Autodesk Inventor part; units mm, degrees
ref_plane "YZ Plane" through (0, 0, 0) normal (1, 0, 0) x (0, 1, 0)
ref_plane "XZ Plane" through (0, 0, 0) normal (0, 1, 0) x (-1, 0, 0)
ref_plane "XY Plane" through (0, 0, 0) normal (0, 0, 1) x (1, 0, 0)
sketch "Sketch1" plane through (0, 0, 0) normal (0, 0, 1) x (1, 0, 0)
  ellipse E0 centre (-7.26, 0) end of major axis (-10.02, 0) minor radius 1.8
  ellipse E1 centre (7.26, 0) end of major axis (10.02, 0) minor radius 1.8
  line L0 (11.52, 0) -> (11.52, 3.95)
  line L1 (11.52, 3.95) -> (15.52, 3.95)
  line L2 (15.52, 3.95) -> (15.52, 9.95)
  line L3 (15.52, 9.95) -> (22.84, 9.95)
  line L4 (22.84, 9.95) -> (22.84, 3.95)
  line L5 (22.84, 3.95) -> (26.84, 3.95)
  line L6 (26.84, 3.95) -> (26.84, 0)
  line L7 (11.52, 0) -> (11.52, -3.95)
  line L8 (11.52, -3.95) -> (15.52, -3.95)
  line L9 (15.52, -3.95) -> (15.52, -9.95)
  line L10 (15.52, -9.95) -> (22.84, -9.95)
  line L11 (22.84, -9.95) -> (22.84, -3.95)
  line L12 (22.84, -3.95) -> (26.84, -3.95)
  line L13 (26.84, -3.95) -> (26.84, 0)
  line L14 (-11.52, 0) -> (-11.52, 3.95)
  line L15 (-11.52, 3.95) -> (-15.52, 3.95)
  line L16 (-15.52, 3.95) -> (-15.52, 9.95)
  line L17 (-15.52, 9.95) -> (-22.84, 9.95)
  line L18 (-22.84, 9.95) -> (-22.84, 3.95)
  line L19 (-22.84, 3.95) -> (-26.84, 3.95)
  line L20 (-26.84, 3.95) -> (-26.84, 0)
  line L21 (-11.52, 0) -> (-11.52, -3.95)
  line L22 (-11.52, -3.95) -> (-15.52, -3.95)
  line L23 (-15.52, -3.95) -> (-15.52, -9.95)
  line L24 (-15.52, -9.95) -> (-22.84, -9.95)
  line L25 (-22.84, -9.95) -> (-22.84, -3.95)
  line L26 (-22.84, -3.95) -> (-26.84, -3.95)
  line L27 (-26.84, -3.95) -> (-26.84, 0)
  circle A0 centre (0, -18) radius 8.5
  circle A1 centre (14.5, -29.5) radius 1.5
  circle A2 centre (-14.5, -29.5) radius 1.5
  circle A3 centre (15, -41.5) radius 2
  circle A4 centre (34, -41.5) radius 2
  circle A5 centre (-15, -41.5) radius 2
  circle A6 centre (-34, -41.5) radius 2
  circle A7 centre (-15, -65.5) radius 2
  circle A8 centre (15, -65.5) radius 2
  circle A9 centre (44, -50.5) radius 1.5
  circle A10 centre (-44, -50.5) radius 1.5
  circle A11 centre (0, -57) radius 1.5
  circle A12 centre (20, -57) radius 1.5
  circle A13 centre (34, -57) radius 1.5
  circle A14 centre (-20, -57) radius 1.5
  circle A15 centre (-34, -57) radius 1.5
  circle A16 centre (23.5, -63) radius 1.5
  circle A17 centre (-23.5, -63) radius 1.5
  line L28 (23.84, 13.95) -> (20.76, 13.95)
  line L29 (20.76, 13.95) -> (20.76, 25.98)
  line L30 (20.76, 25.98) -> (23.84, 25.98)
  line L31 (23.84, 25.98) -> (23.84, 13.95)
  line L32 (-23.84, 13.95) -> (-20.76, 13.95)
  line L33 (-20.76, 13.95) -> (-20.76, 25.98)
  line L34 (-20.76, 25.98) -> (-23.84, 25.98)
  line L35 (-23.84, 25.98) -> (-23.84, 13.95)
  circle A18 centre (15, 37) radius 2
  circle A19 centre (15, 62) radius 2
  circle A20 centre (-15, 37) radius 2
  circle A21 centre (-15, 62) radius 2
  circle A22 centre (35, 41.5) radius 1.5
  circle A23 centre (43.5, 50.5) radius 1.5
  circle A24 centre (-35, 41.5) radius 1.5
  circle A25 centre (-43.5, 50.5) radius 1.5
  circle A26 centre (8.5, 55) radius 1.5
  circle A27 centre (23, 55) radius 1.5
  circle A28 centre (-8.5, 55) radius 1.5
  circle A29 centre (-23, 55) radius 1.5
  circle A30 centre (33, 59) radius 1.5
  circle A31 centre (-33, 59) radius 1.5
  circle A32 centre (24, 62) radius 1.5
  circle A33 centre (-24, 62) radius 1.5
  line L36 (-45, 0) -> (-45, 13.95)
  line L37 (-45, 13.95) -> (-41.92, 13.95)
  line L38 (-41.92, 13.95) -> (-41.92, 25.98)
  line L39 (-41.92, 25.98) -> (-45, 25.98)
  line L40 (-45, 25.98) -> (-45, 38.75)
  line L41 (-45, 38.75) -> (-54.4375, 38.75)
  line L42 (-45, 0) -> (-45, -38.75)
  line L43 (-45, -38.75) -> (-54.4375, -38.75)
  line L44 (45, 0) -> (45, 13.95)
  line L45 (45, 13.95) -> (41.92, 13.95)
  line L46 (41.92, 13.95) -> (41.92, 25.98)
  line L47 (41.92, 25.98) -> (45, 25.98)
  line L48 (45, 25.98) -> (45, 38.75)
  line L49 (45, 38.75) -> (54.4375, 38.75)
  line L50 (45, 0) -> (45, -38.75)
  line L51 (45, -38.75) -> (54.4375, -38.75)
  arc A34 (-56.0386, -41.9485) -> (56.0386, -41.9485) centre (0, 0) ccw
  arc A35 (56.0386, 41.9485) -> (-56.0386, 41.9485) centre (0, 0) ccw
  arc A36 (-56.0386, 41.9485) -> (-54.4375, 38.75) centre (-54.4375, 40.75) ccw
  arc A37 (54.4375, 38.75) -> (56.0386, 41.9485) centre (54.4375, 40.75) ccw
  arc A38 (56.0386, -41.9485) -> (54.4375, -38.75) centre (54.4375, -40.75) ccw
  arc A39 (-54.4375, -38.75) -> (-56.0386, -41.9485) centre (-54.4375, -40.75) ccw
  point P0 (-58.2961, 38.75)
  point P1 (-58.2961, -38.75)
  point P2 (58.2961, 38.75)
  point P3 (58.2961, -38.75)
  dimension "d148" = 2
extrude "Extrusion1" add sketch "Sketch1" along normal blind 2.4
properties part number "Part2_Estructura pequeña"
Input: part model. Units: mm. Frame: model coordinates. Give positions to 0.01 mm unless a question says otherwise; leave off trailing zeros. Loops run counter-clockwise (first coordinate to the right, second up) from the corner with the lowest first, then second, coordinate; pieces in that order, holes last. Notation, with made-up numbers: (-25.5, -39.5) -> (-21.5, -39.5) arc R15 cw to (-21.5, -25.5) -> close; hole circle Ø2 at (38, 69). An arc over 180 degrees is marked (long way). Answer as a JSON object with one key per item and string values. Group by question number.
Item 1: Cut plane C-C, the plane y = -21. Return the cut outline in (x, z).
Item 2: Pull-direction query (Y, two-part tool) for faces 1 (the cylindrical face through (-34.11, 57.99, 1.18)), 2 (the flat face through (-1, 1, 0)); classes: released by +Y, released by -Y, zero draft, split by the parting line, or undercut.
Item 3: Cut plane B-B, the plane z = 1.75. State how many separate pieces and enclosed holes the cut face has, and give its area (3 significant figures).
Item 4: Cut plane D-D, the plane y = 31.5. Return the cut outline in (x, z), and give its area (3 significant figures).
Item 5: Cut plane A-A, the plane y = -5.5. Return the cut outline in (x, z).
Item 6: Line query: probe 1 along Y at (x, z) = (20, 1.6); probe 2 along X at (y, z) = (-40.5, 2.2); probe 3 along Y at (x, z) = (6, 1.9). Output: solid intervals per line, ascending.
Item 7: Pin query (flat end, axial travel): P1, Ø1, axis at x = 33.5, z = 2, coming from the +Y side; P2, Ø0.7, axis at y = 21, z = 1, coming from the -X side; P3, Ø3.5, axis at x = 24, y = 62, coming from the -Z side; P4, Ø1.2, axis at x = 13, z = 1, coming from the +Y side. Return the tip coordinate at first contact, or that it passes through.
Checks:
{
 "1": {"outline": "(-45, 0) -> (-7.95, 0) -> (-7.95, 2.4) -> (-45, 2.4) -> close; (7.95, 0) -> (45, 0) -> (45, 2.4) -> (7.95, 2.4) -> close"},
 "2": {"face 1": "undercut", "face 2": "zero draft"},
 "3": {"separate pieces": "1", "enclosed holes": "40", "area": "11,000 mm²"},
 "4": {"outline": "(-45, 0) -> (45, 0) -> (45, 2.4) -> (-45, 2.4) -> close", "area": "216 mm²"},
 "5": {"outline": "(-45, 0) -> (-22.84, 0) -> (-22.84, 2.4) -> (-45, 2.4) -> close; (-15.52, 0) -> (15.52, 0) -> (15.52, 2.4) -> (-15.52, 2.4) -> close; (22.84, 0) -> (45, 0) -> (45, 2.4) -> (22.84, 2.4) -> close"},
 "6": {"probe 1": "y = -67.08 to -58.5, -55.5 to -9.95, 9.95 to 67.08", "probe 2": "x = -56.42 to -35.73, -32.27 to -16.73, -13.27 to 13.27, 16.73 to 32.27, 35.73 to 56.42", "probe 3": "y = -69.74 to -24.02, -11.98 to -1.6, 1.6 to 69.74"},
 "7": {"P1": "stops at y = 61.73", "P2": "stops at x = -41.92", "P3": "stops at z = 0", "P4": "stops at y = 68.89"}
}
